The figure shows three views and two pictorial views of one solid part (mm, origin at its lowest corner). Answer the questions. A direction names the side the tool comes from. Round coordinates to 2 decimals unless told otherwise and drop trailing zeros. Order: outer loops, then holes, each group sorted by start corner. A loop starts at its lowest first (then second) coordinate and runs counter-clockwise, first axis right, second up. Notation, with made-up numbers: (69, -22.75) - (78, -22.75) arc R18 cw to (78, -2.75) - close; hole circle Ø6 at (22.25, 47). An arc over 180 degrees is marked (long way). Write item = value, one per line.
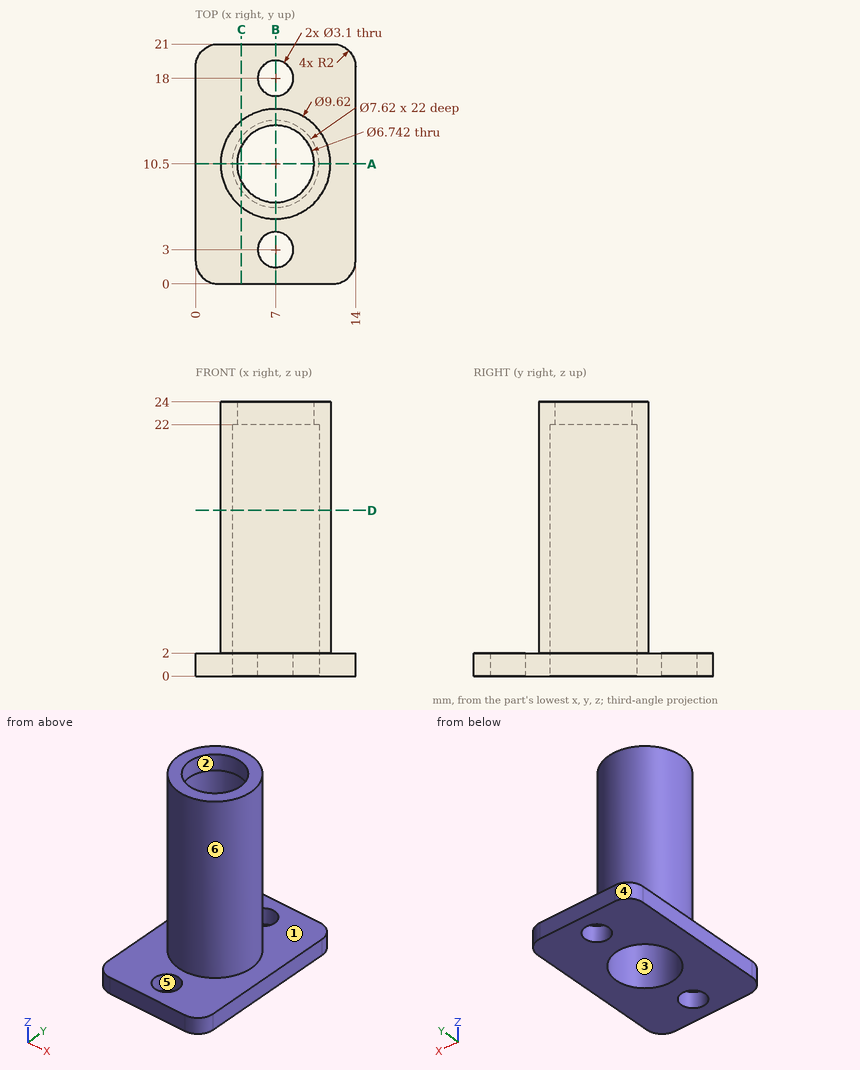
Q1. For the marked faces 1, 2 and 3, determine the directions among +Z, -Z, +X, -X, +Y, -Y from which every point of the face is accessible in a straight line to the end or side of a thin tool.
Model answer:
face_1 = +Z
face_2 = +Z, -Z
face_3 = -Z
Q2. Flat-ended cylindrical pins translate along their axes: P1, Ø1, axis at x = 11.5, z = 9, coming from the +Y side; P2, Ø6, axis at y = 7, z = 21, coming from the +X side; P3, Ø4, axis at x = 9.5, z = 13.5, coming from the +Y side. Find the tip coordinate at first contact, or state that the pin passes through.
Model answer:
P1 = 13.17
P2 = 11.78
P3 = 15.28
Q3. Find the intervals of material crossed by line 1 (Y direction, x = 7, z = 0.75); line 2 (Y direction, x = 7, z = 23.4); line 3 (X direction, y = 3, z = 1), in increasing order. Write a range as from..to.
Model answer:
line_1 = 0..1.45, 4.55..6.69, 14.31..16.45, 19.55..21
line_2 = 5.69..7.13, 13.87..15.31
line_3 = 0..5.45, 8.55..14
Q4. Section D-D on z = 14.5 is taken. Determine the outline of the cut face in (x, y).
Model answer:
outline = circle Ø9.62 at (7, 10.5); hole circle Ø7.62 at (7, 10.5)
Q5. Section C-C on x = 4 is taken. Determine the outline of the cut face in (y, z).
Model answer:
outline = (0, 0) - (8.15, 0) - (8.15, 22) - (8.96, 22) - (8.96, 24) - (6.74, 24) - (6.74, 2) - (0, 2) - close; (12.04, 22) - (12.85, 22) - (12.85, 0) - (21, 0) - (21, 2) - (14.26, 2) - (14.26, 24) - (12.04, 24) - close
Q6. Section B-B on x = 7 is taken. Determine the outline of the cut face in (y, z).
Model answer:
outline = (0, 0) - (1.45, 0) - (1.45, 2) - (0, 2) - close; (4.55, 0) - (6.69, 0) - (6.69, 22) - (7.13, 22) - (7.13, 24) - (5.69, 24) - (5.69, 2) - (4.55, 2) - close; (13.87, 22) - (14.31, 22) - (14.31, 0) - (16.45, 0) - (16.45, 2) - (15.31, 2) - (15.31, 24) - (13.87, 24) - close; (19.55, 0) - (21, 0) - (21, 2) - (19.55, 2) - close
Q7. Section A-A on y = 10.5 is taken. Determine the outline of the cut face in (x, z).
Model answer:
outline = (0, 0) - (3.19, 0) - (3.19, 22) - (3.63, 22) - (3.63, 24) - (2.19, 24) - (2.19, 2) - (0, 2) - close; (10.37, 22) - (10.81, 22) - (10.81, 0) - (14, 0) - (14, 2) - (11.81, 2) - (11.81, 24) - (10.37, 24) - close
Q8. Determine the mould class of the marked faces 4, 5 and 6 for opening direction X: released by +X, released by -X, zero draft, split by the parting line, or undercut.
Model answer:
face_4 = released by -X
face_5 = undercut
face_6 = split by the parting line
